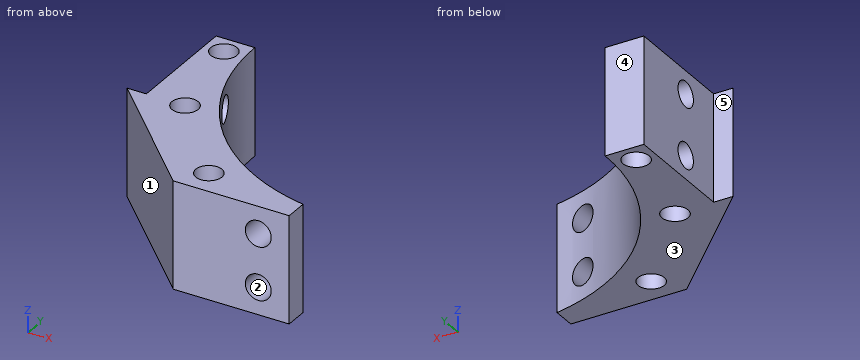
from build123d import *

# Parameters (mm, degrees)
SKETCH_1_W          = 30
SKETCH_1_H          = 30
SKETCH_1_W_2        = 25
EXTRUDE_1_DEPTH     = 27.7
SKETCH_3_R          = 55
CUT_EXTRUDE_1_DEPTH = 40
SKETCH_4_R          = 3.4
CUT_EXTRUDE_2_DEPTH = 90.259677346
SKETCH_5_R          = 3.3
CUT_EXTRUDE_3_DEPTH = 86.978427527
SKETCH_6_R          = 3.35
CUT_EXTRUDE_4_DEPTH = 90.259677512


with BuildPart() as part:
    # 草图1 → 凸台-拉伸1 (new body)
    with BuildSketch(Plane.XY):
        Polygon((0, 30), (30, 0), (30, 30), align=None)
        with Locations((45, 15)):
            Rectangle(SKETCH_1_W, SKETCH_1_H)
        with Locations((17.5, 45)):
            Rectangle(SKETCH_1_W_2, SKETCH_1_H)
    extrude(amount=EXTRUDE_1_DEPTH)

    # 草图3 → 切除-拉伸1 (cut)
    with BuildSketch(Plane.XY.offset(27.7)):
        with Locations((70, 60)):
            Circle(SKETCH_3_R)
    extrude(amount=-CUT_EXTRUDE_1_DEPTH, mode=Mode.SUBTRACT)

    # 草图4 → 切除-拉伸2 (cut, through all)
    with BuildSketch(Plane.XY.offset(27.7)):
        with Locations((35, 7)):
            Circle(SKETCH_4_R)
        with Locations((10, 55)):
            Circle(SKETCH_4_R)
        with Locations((15, 30)):
            Circle(SKETCH_4_R)
    extrude(amount=-CUT_EXTRUDE_2_DEPTH, mode=Mode.SUBTRACT)

    # 草图5 → 切除-拉伸3 (cut, through all)
    with BuildSketch(Plane.ZY.offset(-5)):
        with Locations(Location((6, 42, 0), (0, 0, 270))):
            Circle(SKETCH_5_R)
        with Locations(Location((21.7, 42, 0), (0, 0, 270))):
            Circle(SKETCH_5_R)
    extrude(amount=-CUT_EXTRUDE_3_DEPTH, mode=Mode.SUBTRACT)

    # 草图6 → 切除-拉伸4 (cut, through all)
    with BuildSketch(Plane.XZ):
        with Locations(Location((52, 20.7, 0), (0, 0, 270))):
            Circle(SKETCH_6_R)
        with Locations(Location((52, 7, 0), (0, 0, 270))):
            Circle(SKETCH_6_R)
    extrude(amount=-CUT_EXTRUDE_4_DEPTH, mode=Mode.SUBTRACT)


solid = part.part
Could you check a few things on this model? Use its own coordinates, in mm. Face numbers are marked on the shaded views. A direction names the side the tool comes from. Round coordinates to 2 decimals unless told otherwise and drop trailing zeros. Write each loop counter-clockwise with the first axis right and the second up, starting at its lowest first coordinate (ties: lowest second). Pieces come first, ordered by that corner, then holes. Notation, with made-up numbers: (-21.5, -19.5) -> (-7.5, -19.5) arc R12 ccw to (-7.5, -3.5) -> close; hole circle Ø11 at (70.25, 52.5). An arc over 180 degrees is marked (long way). Use a Markdown table: item, result.
1. Which directions (+Z, -Z, +X, -X, +Y, -Y) give clear straight access to the entire face, cutting with the end or side of a thin tool? Please do the marked faces 4 and 5.
Answer key:
| item | result |
|---|---|
| face 4 | +Z, -Z, +X, -X, +Y |
| face 5 | +Z, -Z, -X, +Y |
2. For pin 1 Ø8 at (y, z) = (14, 20) entering from +X; pin 2 Ø6 at (x, z) = (50, 4) entering from +Y; pin 3 Ø3 at (y, z) = (26.5, 20.5) entering from +X, each with a flat end and sliding along its axis, tell me the tip position at first contact or that it passes through.
Answer key:
| item | result |
|---|---|
| pin 1 | stops at x = 47.09 |
| pin 2 | stops at y = 10.04 |
| pin 3 | stops at x = 27.57 |
3. If we section it at B-B (z = 21.7): List the corners of the cut face in (x, y) for me, then the cut area to 3 significant figures.
Answer key:
| item | result |
|---|---|
| outline | (0, 30) -> (30, 0) -> (48.8, 0) -> (48.8, 9.25) arc R55 cw to (19.29, 38.7) -> (5, 38.7) -> (5, 30) -> close; (5, 45.3) -> (17, 45.3) arc R55 cw to (15, 60) -> (5, 60) -> close; (55.2, 0) -> (60, 0) -> (60, 5.92) arc R55 cw to (55.2, 7.03) -> close; hole circle Ø6.8 at (10, 55); hole circle Ø6.8 at (15, 30); hole circle Ø6.8 at (35, 7) |
| area | 924 mm^2 |
4. If we section it at D-D (z = 15.25): List the corners of the cut face in (x, y) for me, then the cut area to 3 significant figures.
Answer key:
| item | result |
|---|---|
| outline | (0, 30) -> (30, 0) -> (60, 0) -> (60, 5.92) arc R55 cw to (15, 60) -> (5, 60) -> (5, 30) -> close; hole circle Ø6.8 at (10, 55); hole circle Ø6.8 at (15, 30); hole circle Ø6.8 at (35, 7) |
| area | 1,060 mm^2 |
5. Please list where these lines run through material, in increasing order: probe 1 along Y at (x, z) = (11.5, 6); probe 2 along Y at (x, z) = (12.5, 6); probe 3 along Y at (x, z) = (37.5, 23.75).
Answer key:
| item | result |
|---|---|
| probe 1 | y = 18.5 to 38.7, 45.3 to 51.95, 58.05 to 60 |
| probe 2 | y = 17.5 to 27.7, 32.3 to 38.7, 45.3 to 52.7, 57.3 to 60 |
| probe 3 | y = 0 to 4.7, 9.3 to 15.63 |
6. We'd pull the mould along Z, two halves only. Please class the marked faces 1, 2 and 3: +Z half, -Z half, draft (parallel to the pull), parting line (faces both ways), or undercut.
Answer key:
| item | result |
|---|---|
| face 1 | draft |
| face 2 | undercut |
| face 3 | -Z half |
7. If we section it at C-C (y = 41): List the corners of the cut face in (x, z) for me, then the cut area to 3 significant figures.
Answer key:
| item | result |
|---|---|
| outline | (5, 0) -> (18.39, 0) -> (18.39, 2.86) -> (5, 2.86) -> close; (5, 9.14) -> (18.39, 9.14) -> (18.39, 18.56) -> (5, 18.56) -> close; (5, 24.84) -> (18.39, 24.84) -> (18.39, 27.7) -> (5, 27.7) -> close |
| area | 202 mm^2 |
8. If we section it at A-A (x = 10): List the corners of the cut face in (y, z) for me.
Answer key:
| item | result |
|---|---|
| outline | (20, 0) -> (51.6, 0) -> (51.6, 27.7) -> (20, 27.7) -> close; (58.4, 0) -> (60, 0) -> (60, 27.7) -> (58.4, 27.7) -> close; hole circle Ø6.6 at (42, 6); hole circle Ø6.6 at (42, 21.7) |
